For this review, take the finished solid that the model builds, in its own axes (mm). A direction names the side the tool comes from. Round coordinates to 2 decimals unless told otherwise and drop trailing zeros. Loops run counter-clockwise (first coordinate to the right, second up) from the corner with the lowest first, then second, coordinate; pieces in that order, holes last.
```python
from build123d import *

# Parameters (mm, degrees)
SKETCH1_R                                      = 1
BOSS_EXTRUDE1_DEPTH                            = 3
CSK_FOR_M2_FLAT_HEAD_MACHINE_SCREW1_AT_2_COUNT = 2
CSK_FOR_M2_FLAT_HEAD_MACHINE_SCREW1_AT_2_PITCH = 13.775
CSK_FOR_M2_FLAT_HEAD_MACHINE_SCREW1_AT_3_COUNT = 2
CSK_FOR_M2_FLAT_HEAD_MACHINE_SCREW1_AT_3_PITCH = 33
CSK_FOR_M2_FLAT_HEAD_MACHINE_SCREW1_AT_4_COUNT = 2
CSK_FOR_M2_FLAT_HEAD_MACHINE_SCREW1_AT_4_PITCH = 35.759622831


with BuildPart() as part:
    # Sketch1 → Boss-Extrude1 (new body)
    with BuildSketch(Plane(origin=(0, 0, 0), x_dir=(1, 0, 0), z_dir=(0, 1, 0))):
        Polygon((-30, 10.5), (-30, -10.5), (-4, -10.5), (-4, -7), (4, -7), (4, -10.5), (30, -10.5), (30, 10.5), (4, 10.5), (4, 7), (-4, 7), (-4, 10.5), align=None)
        with Locations((16.5, -6.8875)):
            Circle(SKETCH1_R, mode=Mode.SUBTRACT)
        with Locations((-16.5, -6.8875)):
            Circle(SKETCH1_R, mode=Mode.SUBTRACT)
        with Locations((-16.5, 6.8875)):
            Circle(SKETCH1_R, mode=Mode.SUBTRACT)
        with BuildLine():
            Line((-25.085786438, 3.275), (-7.914213562, 3.275))
            ThreePointArc((-7.914213562, 3.275), (-6.5, 3.275), (-6.5, 1.860786438))
            Line((-6.5, 1.860786438), (-6.5, -1.860786438))
            ThreePointArc((-6.5, -1.860786438), (-6.5, -3.275), (-7.914213562, -3.275))
            Line((-7.914213562, -3.275), (-25.085786438, -3.275))
            ThreePointArc((-25.085786438, -3.275), (-26.5, -3.275), (-26.5, -1.860786438))
            Line((-26.5, -1.860786438), (-26.5, 1.860786438))
            ThreePointArc((-26.5, 1.860786438), (-26.5, 3.275), (-25.085786438, 3.275))
        make_face(mode=Mode.SUBTRACT)
        with Locations((16.5, 6.8875)):
            Circle(SKETCH1_R, mode=Mode.SUBTRACT)
        with BuildLine():
            Line((26.5, 1.860786438), (26.5, -1.860786438))
            ThreePointArc((26.5, -1.860786438), (26.5, -3.275), (25.085786438, -3.275))
            Line((25.085786438, -3.275), (7.914213562, -3.275))
            ThreePointArc((7.914213562, -3.275), (6.5, -3.275), (6.5, -1.860786438))
            Line((6.5, -1.860786438), (6.5, 1.860786438))
            ThreePointArc((6.5, 1.860786438), (6.5, 3.275), (7.914213562, 3.275))
            Line((7.914213562, 3.275), (25.085786438, 3.275))
            ThreePointArc((25.085786438, 3.275), (26.5, 3.275), (26.5, 1.860786438))
        make_face(mode=Mode.SUBTRACT)
    extrude(amount=BOSS_EXTRUDE1_DEPTH)

    # Sketch3 → CSK for M2 Flat Head Machine Screw1 (revolve, cut)
    with BuildSketch(Plane(origin=(-16.5, 3, -6.8875), x_dir=(0, 0, 1), z_dir=(1, 0, 0))):
        Polygon((0, 0), (0, 3), (1, 3), (1, 1.2), (2, 0.2), (2, 0), align=None)
    csk_for_m2_flat_head_machine_screw1 = revolve(axis=Axis((-16.5, 9.35, -6.8875), (0, -1, 0)), mode=Mode.SUBTRACT)

    # CSK for M2 Flat Head Machine Screw1 at 2: CSK for M2 Flat Head Machine Screw1 ×2
    with Locations(*[(0, 0, i * CSK_FOR_M2_FLAT_HEAD_MACHINE_SCREW1_AT_2_PITCH) for i in range(1, CSK_FOR_M2_FLAT_HEAD_MACHINE_SCREW1_AT_2_COUNT)]):
        add(csk_for_m2_flat_head_machine_screw1, mode=Mode.SUBTRACT)

    # CSK for M2 Flat Head Machine Screw1 at 3: CSK for M2 Flat Head Machine Screw1 ×2
    with Locations(*[(i * CSK_FOR_M2_FLAT_HEAD_MACHINE_SCREW1_AT_3_PITCH, 0, 0) for i in range(1, CSK_FOR_M2_FLAT_HEAD_MACHINE_SCREW1_AT_3_COUNT)]):
        add(csk_for_m2_flat_head_machine_screw1, mode=Mode.SUBTRACT)

    # CSK for M2 Flat Head Machine Screw1 at 4: CSK for M2 Flat Head Machine Screw1 ×2
    with Locations(*[Vector(0.922828525, 0, 0.385210998) * (i * CSK_FOR_M2_FLAT_HEAD_MACHINE_SCREW1_AT_4_PITCH) for i in range(1, CSK_FOR_M2_FLAT_HEAD_MACHINE_SCREW1_AT_4_COUNT)]):
        add(csk_for_m2_flat_head_machine_screw1, mode=Mode.SUBTRACT)


solid = part.part
```
(1) For faces 5 (the flat face through (4, 1, -9)), 6 (the flat face through (0, 0, 0)), 7 (the flat face through (17, 1, 3.275)), list the 3-axis set-ups (+Z, -Z, +X, -X, +Y, -Y) from which the entire face can be reached by the end or side of a thin tool; tool diameter is ignored.
(2) Insertion check: pin 1 Ø3 at (x, z) = (16.5, -6.89) entering from +Y; pin 2 Ø2.5 at (x, z) = (-16.5, -6.89) entering from +Y; pin 3 Ø1.5 at (x, y) = (0, 2) entering from -Z. Each pin has a flat end and moves straight along its axis. Give the tip position at first contact, or say it passes through.
(3) Add section A-A (z = 1.25). Give the boundary of the cut face in (x, y).
(4) Add section C-C (y = 0.6). Give the number of separate pieces and of enclosed holes in the cut face, plus the area to 3 significant figures.
(5) Add section B-B (x = 13.5). Give the boundary of the cut face in (y, z) (3 decimals), plus the area to 4 significant figures.
(6) The part is to be moulded in two halves that separate along Z. For faces 1 (the flat face through (17, 1, 10.5)), 2 (the flat face through (-16, 1, 3.275)), 3 (the flat face through (0, 1, -7)), 4 (the flat face through (4, 1, 9)), say which applies: pulls with the +Z half, pulls with the -Z half, needs draft (parallel to the pull), parting line crosses it, or undercut.
(7) For L1, parallel to Z at x = -16.5, y = 0.65 (1 decimal); L2, parallel to X at y = 0.4, z = -0.25; L3, parallel to Z at x = 18, y = 0.8 (3 decimals), list the stretches that pass through material, from the lowest coordinate up.
Outcome:
1. face 5: -Z, +Y, -Y
1. face 6: +Z, -Z, +X, -X, -Y
1. face 7: +Y, -Y
2. pin 1: stops at y = 2.3
2. pin 2: stops at y = 2.05
2. pin 3: stops at z = -7
3. outline: (-30, 0) - (-26.5, 0) - (-26.5, 3) - (-30, 3) - close; (-6.5, 0) - (6.5, 0) - (6.5, 3) - (-6.5, 3) - close; (26.5, 0) - (30, 0) - (30, 3) - (26.5, 3) - close
4. separate pieces: 1
4. enclosed holes: 6
4. area: 925 mm2
5. outline: (0, -10.5) - (3, -10.5) - (3, -3.275) - (0, -3.275) - close; (0, 3.275) - (3, 3.275) - (3, 10.5) - (0, 10.5) - close
5. area: 43.35 mm2
6. face 1: pulls with the +Z half
6. face 2: undercut
6. face 3: pulls with the -Z half
6. face 4: needs draft
7. L1: z = -10.5 to -7.9, -5.9 to -3.3, 3.3 to 5.9, 7.9 to 10.5
7. L2: x = -30 to -26.5, -6.5 to 6.5, 26.5 to 30
7. L3: z = -10.5 to -3.275, 3.275 to 10.5
